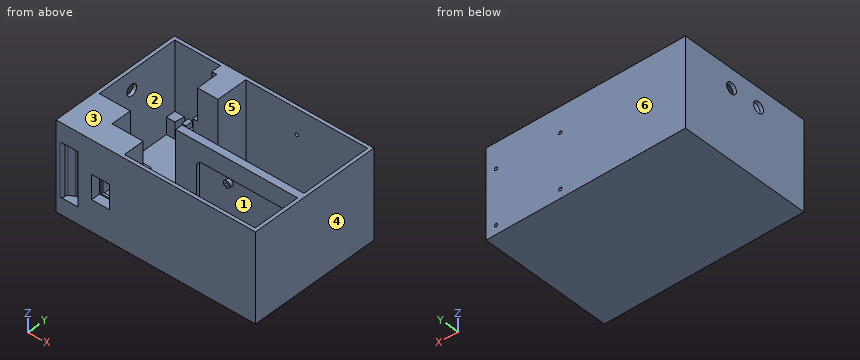
from build123d import *

# Parameters (mm, degrees)
SKETCH1_W                     = 120
SKETCH1_H                     = 180
BOSS_EXTRUDE1_DEPTH           = 80
CUT_EXTRUDE2_DEPTH            = 77
SKETCH5_W                     = 18
SKETCH5_H                     = 28
CUT_EXTRUDE3_DEPTH            = 77
SKETCH7_W                     = 3.814242132
SKETCH7_H                     = 8.503079505
BOSS_EXTRUDE2_DEPTH           = 15
SKETCH8_W                     = 28
SKETCH8_H                     = 12.638642759
CUT_EXTRUDE4_DEPTH            = 62
SKETCH10_W                    = 28
SKETCH10_H                    = 77
BOSS_EXTRUDE5_DEPTH           = 4.8
BOSS_EXTRUDE6_DEPTH           = 15
FILLET1_R                     = 0.5
FILLET2_R                     = 5
CBORE_FOR_M2_SHCS1_AT_2_COUNT = 2
CBORE_FOR_M2_SHCS1_AT_2_PITCH = 58
CBORE_FOR_M2_SHCS1_AT_3_COUNT = 2
CBORE_FOR_M2_SHCS1_AT_3_PITCH = 49
CBORE_FOR_M2_SHCS1_AT_4_COUNT = 2
CBORE_FOR_M2_SHCS1_AT_4_PITCH = 75.927597091
CUT_EXTRUDE8_DEPTH            = 3
CUT_EXTRUDE8_DEPTH_BACK       = 45
FILLET3_R                     = 2
SKETCH21_R                    = 5
CUT_EXTRUDE9_DEPTH            = 25
SKETCH22_W                    = 22
SKETCH22_H                    = 77
BOSS_EXTRUDE7_DEPTH           = 19
SKETCH23_W                    = 13
SKETCH23_H                    = 19.5
CUT_EXTRUDE10_DEPTH           = 30
SKETCH24_W                    = 16
SKETCH24_H                    = 22
CUT_EXTRUDE11_DEPTH           = 8
SKETCH25_W                    = 15.26548048
SKETCH25_H                    = 25.296285881
CUT_EXTRUDE12_DEPTH           = 12
SKETCH26_R                    = 1.5
CUT_EXTRUDE13_DEPTH           = 73
CUT_EXTRUDE14_DEPTH           = 49
CUT_EXTRUDE14_DEPTH_BACK      = 2
SKETCH27_W                    = 3.814242132
SKETCH27_H                    = 15
SKETCH28_W                    = 45.579677418
SKETCH28_H                    = 67.957985629
CUT_EXTRUDE15_DEPTH           = 29
SKETCH29_W                    = 19
SKETCH29_H                    = 77
CUT_EXTRUDE17_DEPTH           = 8
SKETCH30_W                    = 91.153951036
SKETCH30_H                    = 60.622575867
SKETCH30_R                    = 3
CUT_EXTRUDE18_DEPTH           = 3
FILLET4_R                     = 5


with BuildPart() as part:
    # Sketch1 → Boss-Extrude1 (new body)
    with BuildSketch(Plane(origin=(0, 0, 0), x_dir=(0, 1, 0), z_dir=(0, 0, 1))):
        Rectangle(SKETCH1_W, SKETCH1_H)
    extrude(amount=BOSS_EXTRUDE1_DEPTH)

    # Sketch4 → Cut-Extrude2 (cut)
    with BuildSketch(Plane(origin=(-1315.649869597, -737.347167088, 80), x_dir=(1, 0, 0), z_dir=(0, 0, 1))):
        Polygon((1292.649869597, 766.347167088), (1256.649869597, 766.347167088), (1256.649869597, 794.347167088), (1228.649869597, 794.347167088), (1228.649869597, 730.347167088), (1256.649869597, 730.347167088), (1256.649869597, 699.347167088), (1267.649869597, 699.347167088), (1267.649869597, 680.347167088), (1289.649869597, 680.347167088), (1289.649869597, 699.347167088), (1292.649869597, 699.347167088), (1292.649869597, 680.347167088), (1402.649869597, 680.347167088), (1402.649869597, 723.347167088), (1292.649869597, 723.347167088), (1292.649869597, 729.847167088), (1402.649869597, 729.847167088), (1402.649869597, 794.347167088), (1292.649869597, 794.347167088), align=None)
    extrude(amount=-CUT_EXTRUDE2_DEPTH, mode=Mode.SUBTRACT)

    # Sketch5 → Cut-Extrude3 (cut)
    with BuildSketch(Plane(origin=(-1315.649869597, -737.347167088, 80), x_dir=(1, 0, 0), z_dir=(0, 0, 1))):
        with Locations((1265.649869597, 780.347167088)):
            Rectangle(SKETCH5_W, SKETCH5_H)
    extrude(amount=-CUT_EXTRUDE3_DEPTH, mode=Mode.SUBTRACT)

    # Sketch7 → Boss-Extrude2 (add)
    with BuildSketch(Plane.XY.offset(3)):
        Polygon((-66.505568734, 48.496920495), (-59, 48.496920495), (-59, 57), (-67.961780033, 57), align=None)
        Polygon((-59, -7), (-59, 1.503079505), (-66.505568734, 1.503079505), (-67.961780033, -7), align=None)
        with Locations((-73.022462164, -2.748460247)):
            Rectangle(SKETCH7_W, SKETCH7_H)
        with Locations((-73.022462164, 52.748460248)):
            Rectangle(SKETCH7_W, SKETCH7_H)
        Polygon((-87, 57), (-87, 48.496920495), (-79.494431266, 48.496920495), (-78.038219967, 57), align=None)
        Polygon((-79.494431266, 1.503079505), (-87, 1.503079505), (-87, -7), (-77.995952978, -7), align=None)
    extrude(amount=BOSS_EXTRUDE2_DEPTH)

    # Sketch8 → Cut-Extrude4 (cut)
    with BuildSketch(Plane.XY.offset(80)):
        with Locations((-73, -13.319321379)):
            Rectangle(SKETCH8_W, SKETCH8_H)
    extrude(amount=-CUT_EXTRUDE4_DEPTH, mode=Mode.SUBTRACT)

    # Sketch10 → Boss-Extrude5 (add)
    with BuildSketch(Plane(origin=(-41, 0, 0), x_dir=(0, -1, 0), z_dir=(-1, 0, 0))):
        with Locations((-43, 41.5)):
            Rectangle(SKETCH10_W, SKETCH10_H)
    extrude(amount=BOSS_EXTRUDE5_DEPTH)

    # Sketch12 → Boss-Extrude6 (add)
    with BuildSketch(Plane.XY.offset(18)):
        Polygon((-59, -11.981340953), (-62.404767659, -18.250642754), (-69.565878077, -18.250642754), (-74.409105395, -9.838317886), (-87, -9.838317886), (-87, -19.638642759), (-59, -19.638642759), align=None)
    extrude(amount=BOSS_EXTRUDE6_DEPTH)

    # Fillet1
    fillet1_edges = [part.edges().sort_by_distance(p)[0] for p in [
        (-59, -11.981340953, 25.5),
    ]]
    fillet(fillet1_edges, radius=FILLET1_R)

    # Fillet2
    fillet2_edges = [part.edges().sort_by_distance(p)[0] for p in [
        (-62.404767659, -18.250642754, 25.5),
        (-69.565878077, -18.250642754, 25.5),
    ]]
    fillet(fillet2_edges, radius=FILLET2_R)

    # Sketch15 → CBORE for M2 SHCS1 (revolve, cut)
    with BuildSketch(Plane(origin=(81.053987796, -7.5, 57.123857513), x_dir=(0, 0, 1), z_dir=(1, 0, 0))):
        Polygon((0, 0), (0, 7.281118805), (1.3, 6.5), (1.3, 2), (2.2, 2), (2.2, 0.025), (2.225, 0), align=None)
    cbore_for_m2_shcs1 = revolve(axis=Axis((81.053987796, -1.15, 57.123857513), (0, -1, 0)), mode=Mode.SUBTRACT)

    # CBORE for M2 SHCS1 at 2: CBORE for M2 SHCS1 ×2
    with Locations(*[(-i * CBORE_FOR_M2_SHCS1_AT_2_PITCH, 0, 0) for i in range(1, CBORE_FOR_M2_SHCS1_AT_2_COUNT)]):
        add(cbore_for_m2_shcs1, mode=Mode.SUBTRACT)

    # CBORE for M2 SHCS1 at 3: CBORE for M2 SHCS1 ×2
    with Locations(*[(0, 0, -i * CBORE_FOR_M2_SHCS1_AT_3_PITCH) for i in range(1, CBORE_FOR_M2_SHCS1_AT_3_COUNT)]):
        add(cbore_for_m2_shcs1, mode=Mode.SUBTRACT)

    # CBORE for M2 SHCS1 at 4: CBORE for M2 SHCS1 ×2
    with Locations(*[Vector(-0.7638856255460443, 0, -0.6453516491682101) * (i * CBORE_FOR_M2_SHCS1_AT_4_PITCH) for i in range(1, CBORE_FOR_M2_SHCS1_AT_4_COUNT)]):
        add(cbore_for_m2_shcs1, mode=Mode.SUBTRACT)

    # Sketch18 → Cut-Extrude8 (cut, two sides: drawn at the far end of the back side and taken through both)
    with BuildSketch(Plane(origin=(0, 0, 60), x_dir=(0, -1, 0), z_dir=(0, 0, 1)).offset(-CUT_EXTRUDE8_DEPTH_BACK)):
        Polygon((62.758026494, -84.300198527), (62.758026494, -70.435312794), (58.056801253, -70.435312794), (55.726541794, -68.105053334), (52.155556116, -68.105053334), (52.155556116, -78.542615973), (55.726541794, -84.300198527), align=None)
    extrude(amount=CUT_EXTRUDE8_DEPTH + CUT_EXTRUDE8_DEPTH_BACK, mode=Mode.SUBTRACT)

    # Fillet3
    fillet3_edges = [part.edges().sort_by_distance(p)[0] for p in [
        (-84.300198527, -60, 39),
        (-84.300198527, -55.726541794, 39),
        (-70.435312794, -58.056801253, 39),
        (-68.105053334, -52.155556116, 39),
        (-78.542615973, -52.155556116, 39),
    ]]
    fillet(fillet3_edges, radius=FILLET3_R)

    # Sketch21 → Cut-Extrude9 (cut)
    with BuildSketch(Plane(origin=(-90, 0, 0), x_dir=(0, -1, 0), z_dir=(-1, 0, 0))):
        with Locations((14, 62.936860053)):
            Circle(SKETCH21_R)
        with Locations((-13.368287607, 62.936860053)):
            Circle(SKETCH21_R)
    extrude(amount=-CUT_EXTRUDE9_DEPTH, mode=Mode.SUBTRACT)

    # Sketch22 → Boss-Extrude7 (add)
    with BuildSketch(Plane(origin=(0, -57, 0), x_dir=(-1, 0, 0), z_dir=(0, 1, 0))):
        with Locations((37, 41.5)):
            Rectangle(SKETCH22_W, SKETCH22_H)
    extrude(amount=BOSS_EXTRUDE7_DEPTH)

    # Sketch23 → Cut-Extrude10 (cut)
    with BuildSketch(Plane.XZ.offset(60)):
        with Locations((-49.893782672, 39.05711255)):
            Rectangle(SKETCH23_W, SKETCH23_H)
    extrude(amount=-CUT_EXTRUDE10_DEPTH, mode=Mode.SUBTRACT)

    # Sketch24 → Cut-Extrude11 (cut)
    with BuildSketch(Plane.XZ.offset(60)):
        with Locations((-49.893782672, 39.05711255)):
            Rectangle(SKETCH24_W, SKETCH24_H)
    extrude(amount=-CUT_EXTRUDE11_DEPTH, mode=Mode.SUBTRACT)

    # Sketch25 → Cut-Extrude12 (cut)
    with BuildSketch(Plane(origin=(0, -38, 0), x_dir=(-1, 0, 0), z_dir=(0, 1, 0))):
        with Locations((50.082493717, 38.865083442)):
            Rectangle(SKETCH25_W, SKETCH25_H)
    extrude(amount=-CUT_EXTRUDE12_DEPTH, mode=Mode.SUBTRACT)

    # Sketch26 → Cut-Extrude13 (cut)
    with BuildSketch(Plane(origin=(0, -7.5, 0), x_dir=(-1, 0, 0), z_dir=(0, 1, 0))):
        with Locations(Location((-23.053987796, 57.123857513, 0), (0, 0, 270))):
            Circle(SKETCH26_R)
        with Locations(Location((-23.053987796, 8.123857513, 0), (0, 0, 270))):
            Circle(SKETCH26_R)
        with Locations(Location((-81.053987796, 8.123857513, 0), (0, 0, 270))):
            Circle(SKETCH26_R)
        with Locations(Location((-81.053987796, 57.123857513, 0), (0, 0, 270))):
            Circle(SKETCH26_R)
    extrude(amount=CUT_EXTRUDE13_DEPTH, mode=Mode.SUBTRACT)

    # Sketch27 → Cut-Extrude14 (cut, two sides: drawn at the far end of the back side and taken through both)
    with BuildSketch(Plane(origin=(0, 1.503079505, 0), x_dir=(-1, 0, 0), z_dir=(0, 1, 0)).offset(-CUT_EXTRUDE14_DEPTH_BACK)):
        with Locations((73.022462164, 10.5)):
            Rectangle(SKETCH27_W, SKETCH27_H)
    extrude(amount=CUT_EXTRUDE14_DEPTH + CUT_EXTRUDE14_DEPTH_BACK, mode=Mode.SUBTRACT)

    # Sketch28 → Cut-Extrude15 (cut)
    with BuildSketch(Plane.XY.offset(80)):
        with Locations((-64.210161291, 14.340350056)):
            Rectangle(SKETCH28_W, SKETCH28_H)
    extrude(amount=-CUT_EXTRUDE15_DEPTH, mode=Mode.SUBTRACT)

    # Sketch29 → Cut-Extrude17 (cut)
    with BuildSketch(Plane.YZ.offset(-23)):
        with Locations((-47.5, 41.5)):
            Rectangle(SKETCH29_W, SKETCH29_H)
    extrude(amount=-CUT_EXTRUDE17_DEPTH, mode=Mode.SUBTRACT)

    # Sketch30 → Cut-Extrude18 (cut)
    with BuildSketch(Plane.XZ.offset(14)):
        with Locations((41.423024482, 33.311287933)):
            Rectangle(SKETCH30_W, SKETCH30_H)
        with Locations(Location((23.053987796, 8.123857513, 0), (0, 0, 270))):
            Circle(SKETCH30_R, mode=Mode.SUBTRACT)
        with Locations(Location((23.053987796, 57.123857513, 0), (0, 0, 270))):
            Circle(SKETCH30_R, mode=Mode.SUBTRACT)
        with Locations(Location((81.053987796, 8.123857513, 0), (0, 0, 270))):
            Circle(SKETCH30_R, mode=Mode.SUBTRACT)
        with Locations(Location((81.053987796, 57.123857513, 0), (0, 0, 270))):
            Circle(SKETCH30_R, mode=Mode.SUBTRACT)
    extrude(amount=-CUT_EXTRUDE18_DEPTH, mode=Mode.SUBTRACT)

    # Fillet4
    fillet4_edges = [part.edges().sort_by_distance(p)[0] for p in [
        (87, -12.5, 63.622575867),
        (-4.153951036, -12.5, 3),
        (-4.153951036, -12.5, 63.622575867),
    ]]
    fillet(fillet4_edges, radius=FILLET4_R)


solid = part.part
Design review of the part built by this model. Coordinates are the model's own, in mm. Face numbers are marked on the shaded views. A direction names the side the tool comes from. Round coordinates to 2 decimals unless told otherwise and drop trailing zeros. Order: outer loops, then holes, each group sorted by start corner. A loop starts at its lowest first (then second) coordinate and runs counter-clockwise, first axis right, second up.
1) Machinability: for the marked faces 1, 2 and 3, which of the approach directions +Z, -Z, +X, -X, +Y, -Y give a long, thin tool a straight path to every point of the face, cutting with its end or side? Answer none if there is none.
The answers:
face 1: none
face 2: +Z
face 3: +Z, +X, -X, +Y, -Y
2) Consider section D-D (x = 40.5). State the section outline as (y, z) points.
The answers:
outline: (-60, 0) - (60, 0) - (60, 80) - (57, 80) - (57, 3) - (-7.5, 3) - (-7.5, 80) - (-14, 80) - (-14, 63.62) - (-11, 63.62) - (-11, 3) - (-57, 3) - (-57, 80) - (-60, 80) - close
3) Consider section A-A (y = -33). State the section outline as (x, z) points.
The answers:
outline: (-90, 0) - (90, 0) - (90, 80) - (87, 80) - (87, 3) - (-59, 3) - (-59, 80) - (-90, 80) - close
4) Consider section C-C (y = 15). State the section outline as (x, z) points, plus the area to 3 significant figures.
The answers:
outline: (-90, 0) - (90, 0) - (90, 80) - (87, 80) - (87, 3) - (-87, 3) - (-87, 58.21) - (-90, 58.21) - close; (-90, 67.66) - (-87, 67.66) - (-87, 80) - (-90, 80) - close
area: 974 mm2
5) For L1, parallel to X at y = 30, z = 74; L2, parallel to Y at x = -5.5, z = 47.5; L3, parallel to Y at x = 71, z = 61, list the stretches that pass through material, from the lowest coordinate up.
The answers:
L1: x = -90 to -87, -41.42 to -23, 87 to 90
L2: y = -60 to -57, -14 to -7.5, 57 to 60
L3: y = -60 to -57, -11 to -7.5, 57 to 60
6) Draft analysis for pull direction Y (two halves, no side actions). For the marked faces 4, 5 and 6, state which applies: released by +Y, released by -Y, zero draft, split by the parting line, or undercut.
The answers:
face 4: zero draft
face 5: undercut
face 6: released by +Y
7) Consider section B-B (x = -16). State the section outline as (y, z) points, plus the area to 3 significant figures.
The answers:
outline: (-60, 0) - (60, 0) - (60, 80) - (57, 80) - (57, 3) - (-7.5, 3) - (-7.5, 80) - (-14, 80) - (-14, 3) - (-57, 3) - (-57, 80) - (-60, 80) - close
area: 1,320 mm2
8) Clearance check with flat-ended pins moving along their axes: pin 1 Ø5 at (x, y) = (-75, -16) entering from +Z; pin 2 Ø4 at (x, y) = (66, -37.5) entering from +Z; pin 3 Ø2.5 at (x, z) = (23.05, 8.12) entering from +Y. State where each tip first meets the part, or that it passes through.
The answers:
pin 1: stops at z = 33
pin 2: stops at z = 3
pin 3: stops at y = -57
